Check sheet for the modelled part. Datum: model origin and axes. Units: mm. Face numbers are marked on the shaded views. A direction names the side the tool comes from. Round coordinates to 2 decimals unless told otherwise and drop trailing zeros. Write each loop counter-clockwise with the first axis right and the second up, starting at its lowest first coordinate (ties: lowest second). Pieces come first, ordered by that corner, then holes. Notation, with made-up numbers: (-5, -10) -> (47, -10) arc R17 ccw to (47, 21) -> close; hole circle Ø7 at (-36, 18.5). An arc over 180 degrees is marked (long way). One line per item, written item: value.
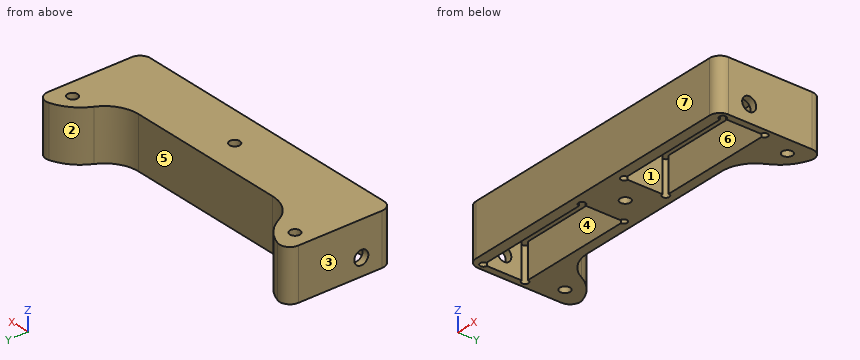
from build123d import *

# Parameters (mm, degrees)
RESSALTO_EXTRUS_O3_DEPTH = 15
CORTE_EXTRUS_O1_DEPTH    = 10.1
ESBO_O3_R                = 1.5
CORTE_EXTRUS_O2_DEPTH    = 16
ESBO_O4_R                = 2.05
CORTE_EXTRUS_O3_DEPTH    = 3
ESBO_O5_R                = 2.05
CORTE_EXTRUS_O4_DEPTH    = 3


with BuildPart() as part:
    # Esboço1 → Ressalto-extrusão3 (new body)
    with BuildSketch(Plane.XY):
        with BuildLine():
            Line((33.436114051, 75.398903013), (-49.563885949, 75.398903013))
            ThreePointArc((-49.563885949, 75.398903013), (-51.685206293, 76.277582669), (-52.563885949, 78.398903013))
            Line((-52.563885949, 78.398903013), (-52.563885949, 93.398903013))
            Line((-52.563885949, 93.398903013), (-52.563885949, 102.938295027))
            ThreePointArc((-52.563885949, 102.938295027), (-51.338709884, 105.356972352), (-48.663885949, 105.800112631))
            ThreePointArc((-48.663885949, 105.800112631), (-44.062022817, 103.23345045), (-40.856925197, 99.051076926))
            ThreePointArc((-40.856925197, 99.051076926), (-37.167666102, 94.929007474), (-31.851570772, 93.398903013))
            Line((-31.851570772, 93.398903013), (-27.063885949, 93.398903013))
            Line((-27.063885949, 93.398903013), (10.936114051, 93.398903013))
            Line((10.936114051, 93.398903013), (15.723798874, 93.398903013))
            ThreePointArc((15.723798874, 93.398903013), (21.039894205, 94.929007474), (24.729153299, 99.051076926))
            ThreePointArc((24.729153299, 99.051076926), (27.934250919, 103.23345045), (32.536114051, 105.800112631))
            ThreePointArc((32.536114051, 105.800112631), (35.210937986, 105.356972352), (36.436114051, 102.938295027))
            Line((36.436114051, 102.938295027), (36.436114051, 93.398903013))
            Line((36.436114051, 93.398903013), (36.436114051, 78.398903013))
            ThreePointArc((36.436114051, 78.398903013), (35.557434395, 76.277582669), (33.436114051, 75.398903013))
        make_face()
    extrude(amount=RESSALTO_EXTRUS_O3_DEPTH)

    # Esboço2 → Corte-extrusão1 (cut)
    with BuildSketch(Plane(origin=(0, 0, 0), x_dir=(-1, 0, 0), z_dir=(0, 0, -1))):
        with BuildLine():
            Line((15.563885949, 89.598903013), (15.563885949, 79.398903013))
            ThreePointArc((15.563885949, 79.398903013), (14.856779168, 77.691796232), (16.563885949, 78.398903013))
            Line((16.563885949, 78.398903013), (49.563885949, 78.398903013))
            ThreePointArc((49.563885949, 78.398903013), (51.27099273, 77.691796232), (50.563885949, 79.398903013))
            Line((50.563885949, 79.398903013), (50.563885949, 89.598903013))
            ThreePointArc((50.563885949, 89.598903013), (51.27099273, 91.306009794), (49.563885949, 90.598903013))
            Line((49.563885949, 90.598903013), (16.563885949, 90.598903013))
            ThreePointArc((16.563885949, 90.598903013), (14.856779168, 91.306009794), (15.563885949, 89.598903013))
        make_face()
        with BuildLine():
            Line((-33.436114051, 90.598903013), (-0.436114051, 90.598903013))
            ThreePointArc((-0.436114051, 90.598903013), (1.27099273, 91.306009794), (0.563885949, 89.598903013))
            Line((0.563885949, 89.598903013), (0.563885949, 79.398903013))
            ThreePointArc((0.563885949, 79.398903013), (1.27099273, 77.691796232), (-0.436114051, 78.398903013))
            Line((-0.436114051, 78.398903013), (-33.436114051, 78.398903013))
            ThreePointArc((-33.436114051, 78.398903013), (-35.143220832, 77.691796232), (-34.436114051, 79.398903013))
            Line((-34.436114051, 79.398903013), (-34.436114051, 89.598903013))
            ThreePointArc((-34.436114051, 89.598903013), (-35.143220832, 91.306009794), (-33.436114051, 90.598903013))
        make_face()
    extrude(amount=-CORTE_EXTRUS_O1_DEPTH, mode=Mode.SUBTRACT)

    # Esboço3 → Corte-extrusão2 (cut, through all)
    with BuildSketch(Plane(origin=(0, 0, 0), x_dir=(-1, 0, 0), z_dir=(0, 0, -1))):
        with Locations((-31.436114051, 99.800112631)):
            Circle(ESBO_O3_R)
        with Locations((47.563885949, 99.800112631)):
            Circle(ESBO_O3_R)
        with Locations((8.063885949, 84.898903013)):
            Circle(ESBO_O3_R)
    extrude(amount=-CORTE_EXTRUS_O2_DEPTH, mode=Mode.SUBTRACT)

    # Esboço4 → Corte-extrusão3 (cut, through all)
    with BuildSketch(Plane.ZY.offset(-34.436114051)):
        with Locations((5, 84.498903013)):
            Circle(ESBO_O4_R)
    extrude(amount=-CORTE_EXTRUS_O3_DEPTH, mode=Mode.SUBTRACT)

    # Esboço5 → Corte-extrusão4 (cut, through all)
    with BuildSketch(Plane(origin=(-50.563885949, 0, 0), x_dir=(0, 0, -1), z_dir=(1, 0, 0))):
        with Locations((-5, 84.498903013)):
            Circle(ESBO_O5_R)
    extrude(amount=-CORTE_EXTRUS_O4_DEPTH, mode=Mode.SUBTRACT)


solid = part.part
Item 1: Mould release check, pull along Y, two halves, no side actions. Record for the marked faces 4, 5, 6 and 7: pulls with the +Y half, pulls with the -Y half, needs draft (parallel to the pull), parting line crosses it, or undercut.
Answer:
face 4: undercut
face 5: pulls with the +Y half
face 6: undercut
face 7: pulls with the -Y half
Item 2: Sectioned sample at D-D on x = -36.5. Enter the section's corners in (y, z).
Answer:
outline: (75.4, 0) -> (78.4, 0) -> (78.4, 10.1) -> (90.6, 10.1) -> (90.6, 0) -> (94.54, 0) -> (94.54, 15) -> (75.4, 15) -> close
Item 3: Thickness scan on line 1 (X direction, y = 90.5, z = 2); line 2 (X direction, y = 99, z = 2); line 3 (X direction, y = 82, z = 9.75). Record the ranges inside material, lowest first.
Answer:
line 1: x = -52.56 to -51.56, -14.57 to -1.56, 35.43 to 36.44
line 2: x = -52.56 to -48.83, -46.3 to -40.83, 24.7 to 30.17, 32.7 to 36.44
line 3: x = -52.56 to -50.56, -15.56 to -0.56, 34.44 to 36.44
Item 4: Sectioned sample at A-A on z = 1.5. Count the separate pieces of the cut face and the enclosed holes in it, and give its area (3 significant figures).
Answer:
separate pieces: 1
enclosed holes: 5
area: 983 mm^2
Item 5: Sectioned sample at B-B on x = 4.5. Enter the section's corners in (y, z), and give its area (3 significant figures).
Answer:
outline: (75.4, 0) -> (78.4, 0) -> (78.4, 10.1) -> (90.6, 10.1) -> (90.6, 0) -> (93.4, 0) -> (93.4, 15) -> (75.4, 15) -> close
area: 147 mm^2
Item 6: Depth check by flat-ended pin: P1, Ø5, axis at x = 14.5, z = 3, coming from the +Y side; P2, Ø1.5, axis at x = 0.5, z = 1.5, coming from the +Y side; P3, Ø1.6, axis at x = -0.56, y = 90.6, coming from the -Z side; P4, Ø2.5, axis at x = 31.44, y = 99.8, coming from the +Z side. Enter the tip coordinate at first touch or a pass-through.
Answer:
P1: stops at y = 93.48
P2: stops at y = 93.4
P3: stops at z = 10.1
P4: passes through
Item 7: Tool access check on the marked faces 1, 2 and 3. Record the directions out of +Z, -Z, +X, -X, +Y, -Y that give a thin tool (end or side, any length) a straight path to the whole face; none if there is none.
Answer:
face 1: -Z
face 2: +Z, -Z, +Y
face 3: +Z, -Z, -X, +Y, -Y
Item 8: Sectioned sample at C-C on z = 13.25. Enter the section's corners in (x, y).
Answer:
outline: (-52.56, 78.4) arc R3 ccw to (-49.56, 75.4) -> (33.44, 75.4) arc R3 ccw to (36.44, 78.4) -> (36.44, 102.94) arc R3 ccw to (32.54, 105.8) arc R13 ccw to (24.73, 99.05) arc R10 cw to (15.72, 93.4) -> (-31.85, 93.4) arc R10 cw to (-40.86, 99.05) arc R13 ccw to (-48.66, 105.8) arc R3 ccw to (-52.56, 102.94) -> close; hole circle Ø3 at (-47.56, 99.8); hole circle Ø3 at (-8.06, 84.9); hole circle Ø3 at (31.44, 99.8)
